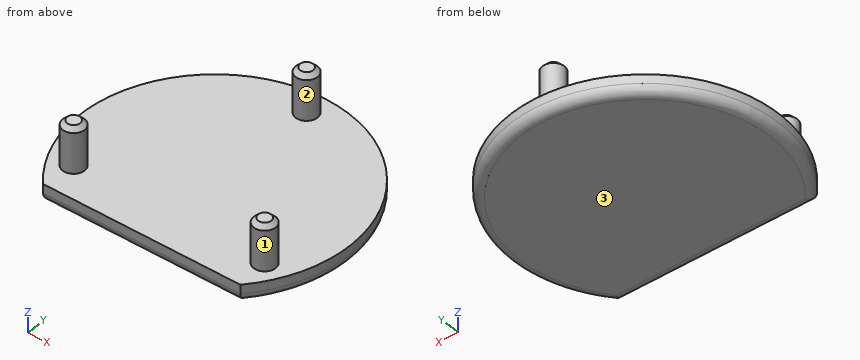
```python
from build123d import *

# Parameters (mm, degrees)
SKETCH_1_R               = 30
EXTRUDE_1_DEPTH          = 4
SKETCH_2_R               = 2.45
EXTRUDE_2_DEPTH          = 10
CUT_EXTRUDE_1_DEPTH      = 45.676615807
CUT_EXTRUDE_1_DEPTH_BACK = 45.676615807
FILLET_1_R               = 2
CHAMFER_1_SIZE           = 1


with BuildPart() as part:
    # 스케치1 → 보스-돌출1 (new body)
    with BuildSketch(Plane.XY):
        Circle(SKETCH_1_R)
    extrude(amount=EXTRUDE_1_DEPTH)

    # 스케치2 → 보스-돌출2 (add)
    with BuildSketch(Plane.XY.offset(4)):
        with Locations((0, 25)):
            Circle(SKETCH_2_R)
        with Locations((21.650635095, -12.5)):
            Circle(SKETCH_2_R)
        with Locations((-21.650635095, -12.5)):
            Circle(SKETCH_2_R)
    extrude(amount=EXTRUDE_2_DEPTH)

    # 스케치3 → 컷-돌출1 (cut, two sides: drawn at the far end of the back side and taken through both)
    with BuildSketch(Plane(origin=(0, 0, 0), x_dir=(-1, 0, 0), z_dir=(0, 0, -1)).offset(-CUT_EXTRUDE_1_DEPTH_BACK)):
        with BuildLine():
            Line((22.360679775, -20), (-22.360679775, -20))
            ThreePointArc((-22.360679775, -20), (0, -30), (22.360679775, -20))
        make_face()
    extrude(amount=CUT_EXTRUDE_1_DEPTH + CUT_EXTRUDE_1_DEPTH_BACK, mode=Mode.SUBTRACT)

    # 필렛1
    fillet_1_edges = [part.edges().sort_by_distance(p)[0] for p in [
        (0, 30, 0),
        (0, -20, 0),
    ]]
    fillet(fillet_1_edges, radius=FILLET_1_R)

    # 모따기1
    chamfer_1_edges = [part.edges().sort_by_distance(p)[0] for p in [
        (-24.100635095, -12.5, 14),
        (-2.45, 25, 14),
        (19.200635095, -12.5, 14),
    ]]
    chamfer(chamfer_1_edges, length=CHAMFER_1_SIZE)


solid = part.part
```
The model under review builds one solid part; all positions refer to its coordinate system, in mm. Face numbers are marked on the shaded views. Give positions to 0.01 mm unless a question says otherwise; leave off trailing zeros. Write each loop counter-clockwise with the first axis right and the second up, starting at its lowest first coordinate (ties: lowest second). Pieces come first, ordered by that corner, then holes.
(1) Consider section B-B, the plane x = 0. Give the boundary of the cut face in (y, z).
(2) To check wall thickness, follow L1, parallel to Z at x = -11, y = -5.5; L2, parallel to Y at x = -25, z = 1; L3, parallel to X at y = 25.5, z = 10.25. State the ranges of each line that lie inside material, in increasing order.
(3) For P1, Ø15, axis at x = -11, y = -3, coming from the +Z side; P2, Ø6, axis at x = 16.5, z = 11.5, coming from the -Y side; P3, Ø5, axis at y = 20.5, z = 8, coming from the -X side, all flat-tipped, find the tip position at first contact; note any pin that passes through.
(4) The part is to be moulded in two halves that separate along X. For the marked faces 1, 2 and 3, say which applies: released by +X, released by -X, zero draft, split by the parting line, or undercut.
(5) Consider section C-C, the plane z = 10. Give the boundary of the cut face in (x, y), and give its area (3 significant figures).
(6) Consider section A-A, the plane y = 0. Give the boundary of the cut face in (x, z), and give its area (3 significant figures).
Returned:
1. outline: (-20, 2) arc R2 ccw to (-18, 0) - (28, 0) arc R2 ccw to (30, 2) - (30, 4) - (27.45, 4) - (27.45, 13) - (26.45, 14) - (23.55, 14) - (22.55, 13) - (22.55, 4) - (-20, 4) - close
2. L1: z = 0 to 4
2. L2: y = -16.09 to 16.09
2. L3: x = -2.4 to 2.4
3. P1: stops at z = 4
3. P2: stops at y = -13.67
3. P3: stops at x = -1.42
4. face 1: undercut
4. face 2: split by the parting line
4. face 3: zero draft
5. outline: circle Ø4.9 at (-21.65, -12.5); circle Ø4.9 at (0, 25); circle Ø4.9 at (21.65, -12.5)
5. area: 56.6 mm2
6. outline: (-30, 2) arc R2 ccw to (-28, 0) - (28, 0) arc R2 ccw to (30, 2) - (30, 4) - (-30, 4) - close
6. area: 238 mm2
